Could you check a few things on this drawing? It's one solid part, dimensions in mm from its lowest x, y, z. A direction names the side the tool comes from. Coordinates: 2 decimals unless noted, no trailing zeros. Loops run counter-clockwise (first coordinate to the right, second up) from the corner with the lowest first, then second, coordinate; pieces in that order, holes last. Notation, with made-up numbers: M 27.25,-35.5 L 45.25,-35.5 A17 ccw 45.25,-31.5 Z; hole C -21,72.25 d10. An arc over 180 degrees is marked long. Answer as a JSON object with one key per item and string values. Group by question number.
Item 1: Suppose I cut it at C-C (x = 16.5). Write out the boundary of the cut face in (y, z) (3 decimals).
Item 2: I'm going to push flat-ended pins straight in: pin 1 Ø3 at (x, y) = (9, 3) entering from -Z; pin 2 Ø5 at (x, z) = (14.5, 16) entering from +Y (3 decimals); pin 3 Ø1 at (y, z) = (4, 11) entering from +X; pin 4 Ø3.5 at (y, z) = (1.5, 20) entering from -X. Where does each tip first touch, or does it pass through?
Item 3: Which directions (+Z, -Z, +X, -X, +Y, -Y) give clear straight access to the entire face, cutting with the end or side of a thin tool? Please do the marked faces 4, 5, 6 and 7.
Item 4: We'd pull the mould along X, two halves only. Please class the marked faces 1, 2 and 3: +X half, -X half, draft (parallel to the pull), parting line (faces both ways), or undercut.
Item 5: Suppose I cut it at D-D (z = 9.25). Write out the boundary of the cut face in (x, y) (3 decimals), then the cut area to 3 significant figures.
Item 6: If I drill on line 1 (Y direction, x = 21.5, z = 15.25) (3 decimals); line 2 (Z direction, x = 2, y = 1) (3 decimals); line 3 (X direction, y = 1, z = 18) (3 decimals), over which ranges is the centre line in solid material (lowest first)?
Item 7: Suppose I cut it at B-B (y = 0.75). Count the separate pieces of the cut face and the enclosed holes in it, then the cut area to 3 significant figures.
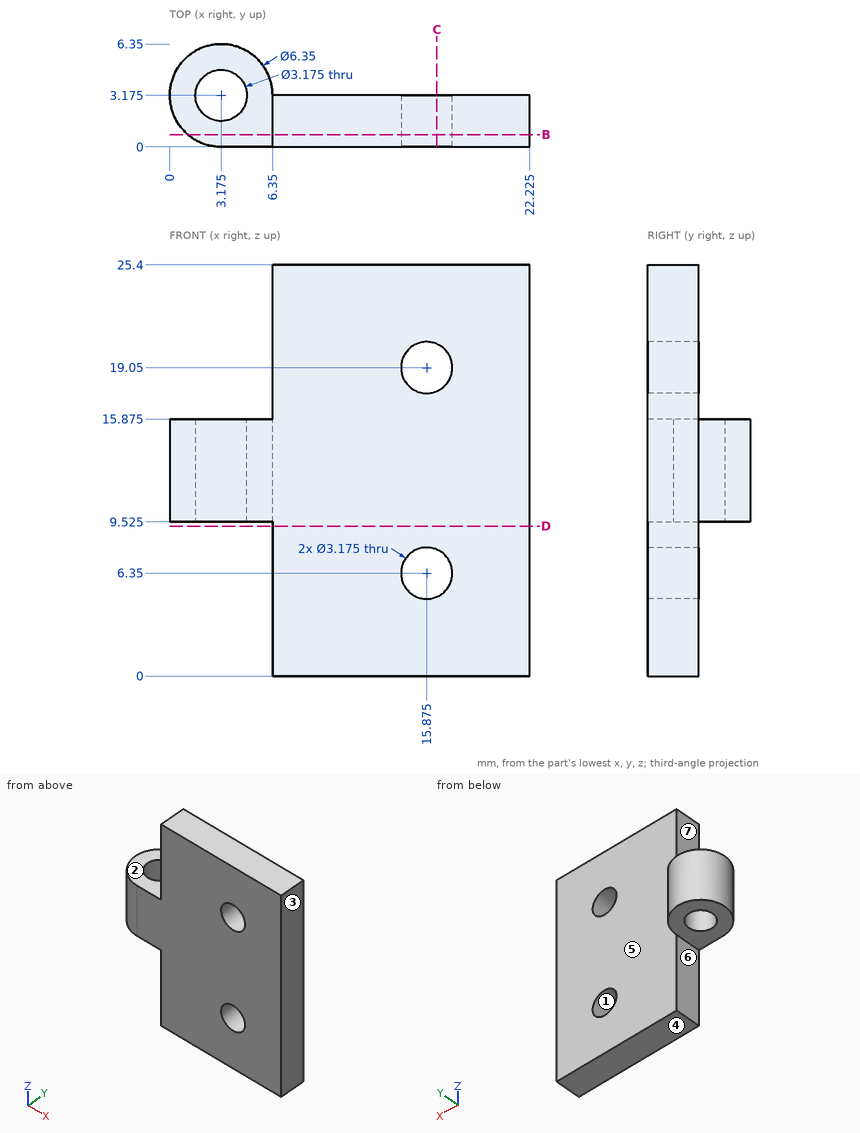
From the geometry:
{
 "1": {"outline": "M 0,0 L 3.175,0 L 3.175,4.891 L 0,4.891 Z; M 0,7.809 L 3.175,7.809 L 3.175,17.591 L 0,17.591 Z; M 0,20.509 L 3.175,20.509 L 3.175,25.4 L 0,25.4 Z"},
 "2": {"pin 1": "z = 0", "pin 2": "y = 3.175", "pin 3": "x = 6.33", "pin 4": "x = 6.35"},
 "3": {"face 4": "-Z, +X, -X, +Y, -Y", "face 5": "+Z, -Z, +X, +Y", "face 6": "-Z, -X, +Y, -Y", "face 7": "+Z, -X, +Y, -Y"},
 "4": {"face 1": "undercut", "face 2": "draft", "face 3": "+X half"},
 "5": {"outline": "M 6.35,0 L 22.225,0 L 22.225,3.175 L 6.35,3.175 Z", "area": "50.4 mm2"},
 "6": {"line 1": "0 to 3.175", "line 2": "9.525 to 15.875", "line 3": "6.35 to 14.684, 17.066 to 22.225"},
 "7": {"separate pieces": "1", "enclosed holes": "2", "area": "421 mm2"}
}
